Build history of the part. All positions in model axes, mm. A direction names the side the tool comes from. Give positions to 0.01 mm unless a question says otherwise; leave off trailing zeros. One line per question, with ' | ' between items. Start each with the question number.
(1) Pull direction Y, two halves, no side cores. Call faces 3 (the face through (25, -115, 5)), 4 (the face through (88.71, -98, 16)), 5 (the face through (2.9, -191, 16)), 6 (the face through (26.109, -113.425, 2.465)): +Y half, -Y half, draft (parallel to the pull), parting line (faces both ways), or undercut.
(2) Pin check, flat tip, straight feed: pin 1 Ø12 at (x, y) = (38, -46) entering from -Z. Stop position of the tip, or through.
(3) Which spindle directions (+Z, -Z, +X, -X, +Y, -Y) get a long thin tool onto all of the face, cutting with end or side? Do faces 1 (the face through (45, 0, 16)), 2 (the face through (63, -115, 5)). Say none if no direction does.
(4) Drill centre lines: L1, parallel to X at y = -114.98, z = 1.45; L2, parallel to Y at x = 25, z = 2; L3, parallel to Y at x = 25.3, z = 2. Where is each one in solid material? Low to high. Write a range as from..to.
from build123d import *

# Parameters (mm, degrees)
F1_DEPTH = 32.51
F2_R     = 1.7525
F3_DEPTH = 5


with BuildPart() as f1:
    # F0 (on Top) → F1 (new body)
    with BuildSketch(Plane.XY):
        with BuildLine():
            Line((78.71, 0), (10, 0))
            ThreePointArc((10, 0), (2.928932, -2.928932), (0, -10))
            Line((0, -10), (0, -183.96))
            ThreePointArc((0, -183.96), (2.928932, -191.031068), (10, -193.96))
            Line((10, -193.96), (78.71, -193.96))
            ThreePointArc((78.71, -193.96), (85.781068, -191.031068), (88.71, -183.96))
            Line((88.71, -183.96), (88.71, -10))
            ThreePointArc((88.71, -10), (85.781068, -2.928932), (78.71, 0))
        make_face()
    extrude(amount=F1_DEPTH)

    # F2 (on face) → F3 (cut)
    with BuildSketch(Plane(origin=(0, 0, 0), x_dir=(1, 0, 0), z_dir=(0, 0, -1))):
        with Locations((63.4, 114.98)):
            Circle(F2_R)
        with Locations((25.3, 114.98)):
            Circle(F2_R)
    extrude(amount=-F3_DEPTH, mode=Mode.SUBTRACT)


solid = f1.part
Result set:
1) face 3: undercut | face 4: draft | face 5: -Y half | face 6: undercut
2) pin 1: stops at z = 0
3) face 1: +Z, -Z, +X, -X, +Y | face 2: -Z
4) L1: x = 0..23.55, 27.05..61.65, 65.15..88.71 | L2: y = -193.96..-116.71, -113.25..0 | L3: y = -193.96..-116.73, -113.23..0
